Here's how the part is built. I have some questions about the finished solid (model axes, mm). A direction names the side the tool comes from. Coordinates: 2 decimals unless noted, no trailing zeros. Write each loop counter-clockwise with the first axis right and the second up, starting at its lowest first coordinate (ties: lowest second). Pieces come first, ordered by that corner, then holes. Notation, with made-up numbers: (14, -9.75) -> (68, -9.75) arc R34 cw to (68, 29.25) -> close; hole circle Ø1 at (-10.5, 52). An arc over 180 degrees is marked (long way). Use a Markdown table: item, result. Add a question column.
Item 1: Imagine slicing it at B-B, the plane z = 5. Write out the boundary of the cut face in (x, y), and give its area (3 significant figures).
Item 2: If I drill on line 1 along X through (y, z) = (-15.75, 37.5); line 2 along X through (y, z) = (-14.75, 5); line 3 along X through (y, z) = (-15, 30), over which ranges is the centre line in solid material (lowest first)? Write a range as from..to.
Item 3: Imagine slicing it at C-C, the plane x = 11.5. Write out the boundary of the cut face in (y, z), and give its area (3 significant figures).
Item 4: On a 3-axis mill with a long thin cutter (end or side, diameter ignored), from which of +Z, -Z, +X, -X, +Y, -Y can I reach the whole of each face in a straight line? I mean faces 4 (the flat face through (6.487, -5, 13)), 5 (the flat face through (7.287, -9, 5)), 6 (the flat face through (11, -5, 16)), 7 (the flat face through (11.3, -6, 2.7)). Say none if no direction works.
Item 5: Imagine slicing it at D-D, the plane x = 4. Write out the boundary of the cut face in (y, z).
Item 6: Will these pins go through, and if not, where does the flat tip stop? pin 1 Ø3 at (y, z) = (-4, 11.5) entering from +X; pin 2 Ø5 at (y, z) = (-4.5, 12) entering from -X; pin 3 Ø3 at (x, y) = (10.5, -5.5) entering from +Z.
Item 7: Imagine slicing it at A-A, the plane y = -12.25. Write out the boundary of the cut face in (x, z).
Item 8: If we mould it in two halves opening along Z, with no side actions, what happens to faces 1 (the flat face through (11, -15, 42)), 2 (the cylindrical face through (12.91, -14.55, 21.01)), 3 (the flat face through (16.087, -5, 13))? For each: pulls with the +Z half, pulls with the -Z half, needs draft (parallel to the pull), parting line crosses it, or undercut.
```python
from build123d import *

# Parameters (mm, degrees)
F0_R      = 1.7
F0_R_2    = 2.1
F0_R_3    = 6.1
F0_W      = 0.8
F0_H      = 6
F1_DEPTH  = 18
F2_W      = 6
F2_H      = 10
F3_DEPTH  = 20.001
F4_DEPTH  = 5.2
F5_W      = 37.3805030249
F5_H      = 33.9431622997
F6_DEPTH  = 6
F7_DEPTH  = 6
F8_W      = 20
F8_H      = 6.8
F9_DEPTH  = 16
F10_DEPTH = 18.001


with BuildPart() as f1:
    # F0 (on Front) → F1 (new body)
    with BuildSketch(Plane.XZ):
        Polygon((1.2868126808, 42), (1.2868126808, 31.58263134), (1.2868126808, 16), (6.4868126808, 16), (7.2868126808, 16), (7.2868126808, 10), (7.2868126808, 0), (15.2868126808, 0), (15.2868126808, 10), (15.2868126808, 16), (16.0868126808, 16), (21.2868126808, 16), (21.2868126808, 31.58263134), (21.2868126808, 42), align=None)
        with Locations((11.2868126808, 20.5)):
            Circle(F0_R, mode=Mode.SUBTRACT)
        with Locations((11.2868126808, 5)):
            Circle(F0_R_2, mode=Mode.SUBTRACT)
        with Locations((11.2868126808, 30)):
            Circle(F0_R_3, mode=Mode.SUBTRACT)
        with Locations((4.7868126808, 37.5)):
            Circle(F0_R, mode=Mode.SUBTRACT)
        with Locations((17.7868126808, 37.5)):
            Circle(F0_R, mode=Mode.SUBTRACT)
        with Locations((6.8868126808, 13)):
            Rectangle(F0_W, F0_H)
        with Locations((15.6868126808, 13)):
            Rectangle(F0_W, F0_H)
    extrude(amount=F1_DEPTH)

    # F2 (on face) → F3 (cut, through all)
    with BuildSketch(Plane.YZ.offset(21.2868126808)):
        with Locations((-3, 5)):
            Rectangle(F2_W, F2_H)
    extrude(amount=-F3_DEPTH, mode=Mode.SUBTRACT)

    # F4 (cut): a face of the model
    f4_faces = [f1.faces().sort_by_distance(p)[0] for p in [
        (20.9094534356, 0, 29),
    ]]
    extrude(f4_faces, amount=-F4_DEPTH, mode=Mode.SUBTRACT)

    # F5 (on face) → F6 (cut)
    with BuildSketch(Plane(origin=(0, -5.2, 0), x_dir=(-1, 0, 0), z_dir=(0, 1, 0))):
        with Locations((-12.0248973835, 32.9715811498)):
            Rectangle(F5_W, F5_H)
    extrude(amount=-F6_DEPTH, mode=Mode.SUBTRACT)

    # F7 (add): a face of the model
    f7_faces = [f1.faces().sort_by_distance(p)[0] for p in [
        (11.2868126808, -5.2, 13),
    ]]
    extrude(f7_faces, amount=F7_DEPTH)

    # F8 (on face) → F9 (join)
    with BuildSketch(Plane(origin=(0, 0, 16), x_dir=(1, 0, 0), z_dir=(0, 0, -1))):
        with Locations((11.2868126808, 14.6)):
            Rectangle(F8_W, F8_H)
    extrude(amount=F9_DEPTH)

    # F0 (on Front) → F10 (cut, through all)
    with BuildSketch(Plane.XZ):
        with Locations((11.2868126808, 5)):
            Circle(F0_R_2)
    extrude(amount=F10_DEPTH, mode=Mode.SUBTRACT)


solid = f1.part
```
Ans:
| question | item | result |
|---|---|---|
| 1 | outline | (1.29, -18) -> (9.19, -18) -> (9.19, -6) -> (7.29, -6) -> (7.29, -11.2) -> (1.29, -11.2) -> close; (13.39, -18) -> (21.29, -18) -> (21.29, -11.2) -> (15.29, -11.2) -> (15.29, -6) -> (13.39, -6) -> close |
| 1 | area | 127 mm^2 |
| 2 | line 1 | x = 1.29..3.09, 6.49..16.09, 19.49..21.29 |
| 2 | line 2 | x = 1.29..9.19, 13.39..21.29 |
| 2 | line 3 | x = 1.29..5.19, 17.39..21.29 |
| 3 | outline | (-18, 0) -> (-6, 0) -> (-6, 2.91) -> (-18, 2.91) -> close; (-18, 7.09) -> (-6, 7.09) -> (-6, 10) -> (0.8, 10) -> (0.8, 16) -> (-11.2, 16) -> (-11.2, 18.81) -> (-18, 18.81) -> close; (-18, 22.19) -> (-11.2, 22.19) -> (-11.2, 23.9) -> (-18, 23.9) -> close; (-18, 36.1) -> (-11.2, 36.1) -> (-11.2, 42) -> (-18, 42) -> close |
| 3 | area | 254 mm^2 |
| 4 | face 4 | +Z, -Z, -X, +Y |
| 4 | face 5 | -Z, -X, +Y |
| 4 | face 6 | +Z, +X, -X, +Y |
| 4 | face 7 | -Z, +X, -X, +Y |
| 5 | outline | (-18, 0) -> (-11.2, 0) -> (-11.2, 35.99) -> (-18, 35.99) -> close; (-18, 39.01) -> (-11.2, 39.01) -> (-11.2, 42) -> (-18, 42) -> close |
| 6 | pin 1 | stops at x = 16.09 |
| 6 | pin 2 | stops at x = 6.49 |
| 6 | pin 3 | stops at z = 16 |
| 7 | outline | (1.29, 0) -> (21.29, 0) -> (21.29, 42) -> (1.29, 42) -> close; hole circle Ø3.4 at (4.79, 37.5); hole circle Ø12.2 at (11.29, 30); hole circle Ø4.2 at (11.29, 5); hole circle Ø3.4 at (11.29, 20.5); hole circle Ø3.4 at (17.79, 37.5) |
| 8 | face 1 | pulls with the +Z half |
| 8 | face 2 | undercut |
| 8 | face 3 | needs draft |
